Model file for the job. Use its own axes, mm. Round coordinates to 2 decimals unless told otherwise and drop trailing zeros. Loops run counter-clockwise (first coordinate to the right, second up) from the corner with the lowest first, then second, coordinate; pieces in that order, holes last. Notation, with made-up numbers: (-31.75, 40) - (-27.75, 40) arc R28 ccw to (-27.75, 63) - close; hole circle Ø6 at (76, 22.25). An arc over 180 degrees is marked (long way). Use one line per item in the form item = value.
from build123d import *

# Parameters (mm, degrees)
F0_W     = 11.45
F0_H     = 25.4
F0_R     = 2.5
F1_DEPTH = 2.5


# Not quite as in the source:
# - a feature names something its author has since deleted; it is built from what else it names


with BuildPart() as f1:
    # F0 (on Top) → F1 (new body)
    with BuildSketch(Plane.XY):
        with Locations((6.975, 73.025)):
            Rectangle(F0_W, F0_H)
        with Locations((7.5, 80.725)):
            Circle(F0_R, mode=Mode.SUBTRACT)
        with Locations((-6.975, 73.025)):
            Rectangle(F0_W, F0_H)
        with Locations((-7.5, 80.725)):
            Circle(F0_R, mode=Mode.SUBTRACT)
        with BuildLine():
            ThreePointArc((-10.5302837094, 53.975), (-6.0950122474, 56.1486377797), (-1.25, 57.1089452627))
            Line((-1.25, 57.1089452627), (-1.25, 60.325))
            Line((-1.25, 60.325), (-12.7, 60.325))
            Line((-12.7, 60.325), (-19.05, 60.325))
            Line((-19.05, 60.325), (-19.05, 53.975))
            Line((-19.05, 53.975), (-10.5302837094, 53.975))
        make_face()
        with BuildLine():
            ThreePointArc((1.25, 57.1089452627), (6.0950122474, 56.1486377797), (10.5302837094, 53.975))
            Line((10.5302837094, 53.975), (19.05, 53.975))
            Line((19.05, 53.975), (19.05, 60.325))
            Line((19.05, 60.325), (12.7, 60.325))
            Line((12.7, 60.325), (1.25, 60.325))
            Line((1.25, 60.325), (1.25, 57.1089452627))
        make_face()
        with BuildLine():
            Line((1.25, 53.975), (10.5302837094, 53.975))
            ThreePointArc((10.5302837094, 53.975), (6.0950122474, 56.1486377797), (1.25, 57.1089452627))
            Line((1.25, 57.1089452627), (1.25, 53.975))
        make_face()
        with BuildLine():
            Line((-1.25, 53.975), (-1.25, 57.1089452627))
            ThreePointArc((-1.25, 57.1089452627), (-6.0950122474, 56.1486377797), (-10.5302837094, 53.975))
            Line((-10.5302837094, 53.975), (-1.25, 53.975))
        make_face()
        with BuildLine():
            Line((-1.25, 25.3692234804), (-1.25, 53.975))
            Line((-1.25, 53.975), (-10.5302837094, 53.975))
            ThreePointArc((-10.5302837094, 53.975), (-19.0443993724, 38.5619010114), (-11.2875107666, 22.7541666667))
            ThreePointArc((-11.2875107666, 22.7541666667), (-6.4036649343, 24.5795255326), (-1.25, 25.3692234804))
        make_face()
        with BuildLine():
            ThreePointArc((11.2875107666, 22.7541666667), (16.9989643817, 29.5012960309), (19.05, 38.1))
            ThreePointArc((19.05, 38.1), (16.785475934, 47.1083460007), (10.5302837094, 53.975))
            Line((10.5302837094, 53.975), (1.25, 53.975))
            Line((1.25, 53.975), (1.25, 25.3692234804))
            ThreePointArc((1.25, 25.3692234804), (6.4036649343, 24.5795255326), (11.2875107666, 22.7541666667))
        make_face()
        with BuildLine():
            ThreePointArc((-11.2875107666, 22.7541666667), (-6.5308415466, 20.204452825), (-1.25, 19.0910547373))
            Line((-1.25, 19.0910547373), (-1.25, 25.3692234804))
            ThreePointArc((-1.25, 25.3692234804), (-6.4036649343, 24.5795255326), (-11.2875107666, 22.7541666667))
        make_face()
        with BuildLine():
            ThreePointArc((1.25, 19.0910547373), (6.5308415466, 20.204452825), (11.2875107666, 22.7541666667))
            ThreePointArc((11.2875107666, 22.7541666667), (6.4036649343, 24.5795255326), (1.25, 25.3692234804))
            Line((1.25, 25.3692234804), (1.25, 19.0910547373))
        make_face()
        with BuildLine():
            ThreePointArc((-18.4450831863, -17.4625), (0, -25.4), (18.4450831863, -17.4625))
            ThreePointArc((18.4450831863, -17.4625), (0, -12.7), (-18.4450831863, -17.4625))
        make_face()
        with BuildLine():
            ThreePointArc((38.1, -50.8), (32.820478892, -31.4499052896), (18.4450831863, -17.4625))
            ThreePointArc((18.4450831863, -17.4625), (0, -25.4), (-18.4450831863, -17.4625))
            ThreePointArc((-18.4450831863, -17.4625), (-19.3500947104, -83.620478892), (38.1, -50.8))
        make_face()
        with BuildLine():
            ThreePointArc((25.4, 0), (21.5854438624, 13.3876291129), (11.2875107666, 22.7541666667))
            ThreePointArc((11.2875107666, 22.7541666667), (6.5308415466, 20.204452825), (1.25, 19.0910547373))
            Line((1.25, 19.0910547373), (1.25, -1.5875))
            Line((1.25, -1.5875), (-1.25, -1.5875))
            Line((-1.25, -1.5875), (-1.25, 19.0910547373))
            ThreePointArc((-1.25, 19.0910547373), (-6.5308415466, 20.204452825), (-11.2875107666, 22.7541666667))
            ThreePointArc((-11.2875107666, 22.7541666667), (-25.0070361146, 4.4506341979), (-18.4450831863, -17.4625))
            ThreePointArc((-18.4450831863, -17.4625), (0, -12.7), (18.4450831863, -17.4625))
            ThreePointArc((18.4450831863, -17.4625), (23.5972997707, -9.3982681135), (25.4, 0))
        make_face()
    extrude(amount=F1_DEPTH)


solid = f1.part
1. Cut at B-B, the plane x = -22. Give the cut face in (y, z).
Geometry check:
outline = (-81.91, 0) - (-19.69, 0) - (-19.69, 2.5) - (-81.91, 2.5) - close; (-12.69, 0) - (12.69, 0) - (12.69, 2.5) - (-12.69, 2.5) - close
2. Flat gauge pins, fed straight in: pin 1 (6 mm diameter, centred on x = -7.5, y = 80.725, fed in from -Z); pin 2 (0.8 mm diameter, centred on x = 0.5, z = 1, fed in from +Y); pin 3 (0.8 mm diameter, centred on x = -13, z = 0.5, fed in from -Y); pin 4 (1.5 mm diameter, centred on x = 29, z = 1.5, fed in from -Y). Where does each tip first touch, or does it go through?
Geometry check:
pin_1 = 0
pin_2 = -1.59
pin_3 = -86.76
pin_4 = -76.36
3. Wall check: probe 1 along X at (y, z) = (1, 0.6); probe 2 along X at (y, z) = (67, 2.2); probe 3 along Y at (x, z) = (16.5, 1.3) (3 decimals). Give the ranges that are in metal, low to high.
Geometry check:
probe_1 = -25.38 to -1.25, 1.25 to 25.38
probe_2 = -12.7 to -1.25, 1.25 to 12.7
probe_3 = -85.142 to 19.311, 28.579 to 47.621, 53.975 to 60.325
4. Pull direction Y, two halves, no side cores. Call faces 1 (the cylindrical face through (-7.825, 83.204, 1.232)), 2 (the flat face through (-1, -20, 2.5)): +Y half, -Y half, draft (parallel to the pull), parting line (faces both ways), or undercut.
Geometry check:
face_1 = undercut
face_2 = draft
5. Cut at A-A, the plane y = 63.5. Give the cut face in (x, z), plus the area to 4 significant figures.
Geometry check:
outline = (-12.7, 0) - (-1.25, 0) - (-1.25, 2.5) - (-12.7, 2.5) - close; (1.25, 0) - (12.7, 0) - (12.7, 2.5) - (1.25, 2.5) - close
area = 57.25 mm^2
6. Cut at D-D, the plane z = 1.25. Give the number of separate pieces and of enclosed holes in the cut face, plus the area to 3 significant figures.
Geometry check:
separate_pieces = 1
enclosed_holes = 2
area = 7,890 mm^2
7. Cut at C-C, the plane x = 16.5. Give the cut face in (y, z) (3 decimals).
Geometry check:
outline = (-85.142, 0) - (19.311, 0) - (19.311, 2.5) - (-85.142, 2.5) - close; (28.579, 0) - (47.621, 0) - (47.621, 2.5) - (28.579, 2.5) - close; (53.975, 0) - (60.325, 0) - (60.325, 2.5) - (53.975, 2.5) - close
